Job drawing, mm, ordinate dimensions from the low corner. One solid piece. A direction names the side the tool comes from. Coordinates: 2 decimals unless noted, no trailing zeros. Write each loop counter-clockwise with the first axis right and the second up, starting at its lowest first coordinate (ties: lowest second). Pieces come first, ordered by that corner, then holes.
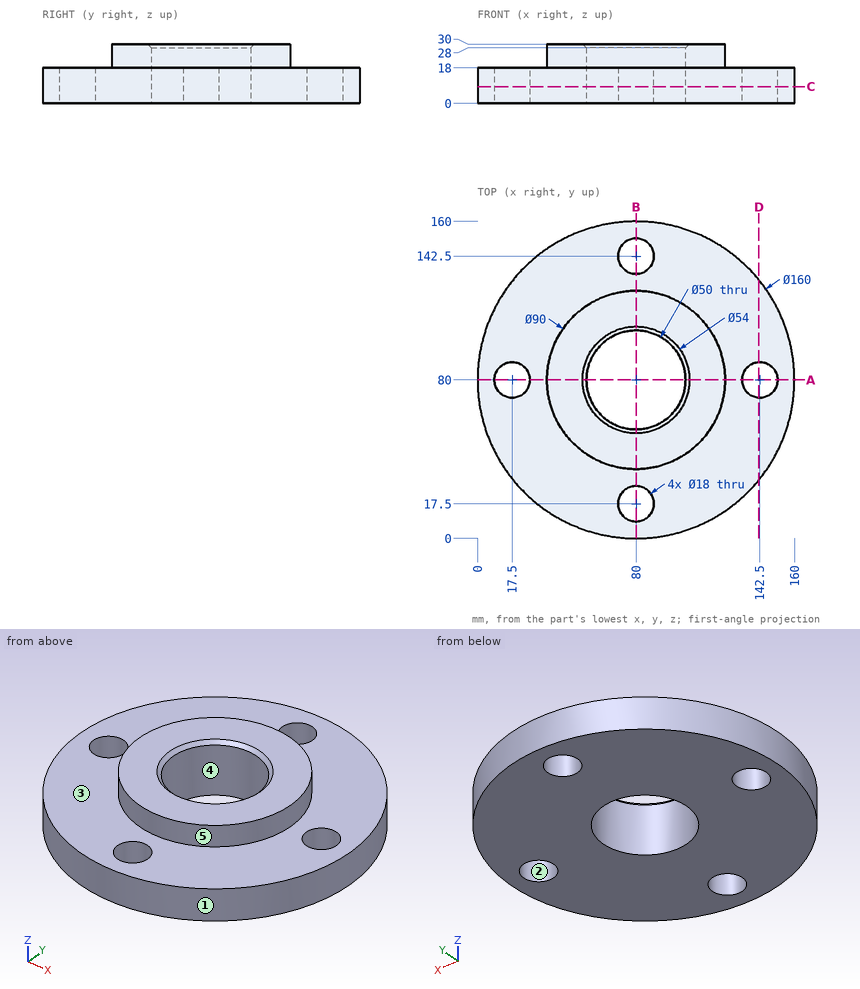
1. Saw through at D-D on x = 142. List the corners of the cut face in (y, z).
Computed values:
outline: (29.44, 0) - (71.01, 0) - (71.01, 18) - (29.44, 18) - close; (88.99, 0) - (130.56, 0) - (130.56, 18) - (88.99, 18) - close
2. Saw through at C-C on z = 8.5. List the corners of the cut face in (x, y), plus the area to 3 significant figures.
Computed values:
outline: circle Ø160 at (80, 80); hole circle Ø18 at (17.5, 80); hole circle Ø50 at (80, 80); hole circle Ø18 at (80, 17.5); hole circle Ø18 at (80, 142.5); hole circle Ø18 at (142.5, 80)
area: 17,100 mm2
3. Probe line 1 along Y through (x, z) = (80, 5.25); line 2 along X through (y, z) = (84, 4.5); line 3 along X through (y, z) = (74.5, 8.5). List the from-to ranges inside material, lowest first.
Computed values:
line 1: y = 0 to 8.5, 26.5 to 55, 105 to 133.5, 151.5 to 160
line 2: x = 0.1 to 9.44, 25.56 to 55.32, 104.68 to 134.44, 150.56 to 159.9
line 3: x = 0.19 to 10.38, 24.62 to 55.61, 104.39 to 135.38, 149.62 to 159.81
4. Flat gauge pins, fed straight in: pin 1 (8 mm diameter, centred on x = 25, y = 49.5, fed in from +Z); pin 2 (10 mm diameter, centred on y = 131.5, z = 8.5, fed in from +X); pin 3 (14.5 mm diameter, centred on x = 17.5, y = 80, fed in from +Z); pin 4 (4 mm diameter, centred on x = 115, z = 7, fed in from +Y). Where does each tip first touch, or does it go through?
Computed values:
pin 1: stops at z = 18
pin 2: stops at x = 145.1
pin 3: passes through
pin 4: stops at y = 152.88
5. 3-axis set-ups, long thin cutter, end or side, ignore diameter. For the marked faces 4 and 5: which of +Z, -Z, +X, -X, +Y, -Y reach the whole face in a straight line?
Computed values:
face 4: +Z, -Z
face 5: +Z
6. Mould opens along X. For the marked faces 1, 2 and 3 say: +X half, -X half, draft (parallel to the pull), parting line (faces both ways), or undercut.
Computed values:
face 1: parting line
face 2: undercut
face 3: draft
7. Saw through at A-A on y = 80. List the corners of the cut face in (x, z).
Computed values:
outline: (0, 0) - (8.5, 0) - (8.5, 18) - (0, 18) - close; (26.5, 0) - (55, 0) - (55, 28) - (53, 30) - (35, 30) - (35, 18) - (26.5, 18) - close; (105, 0) - (133.5, 0) - (133.5, 18) - (125, 18) - (125, 30) - (107, 30) - (105, 28) - close; (151.5, 0) - (160, 0) - (160, 18) - (151.5, 18) - close
